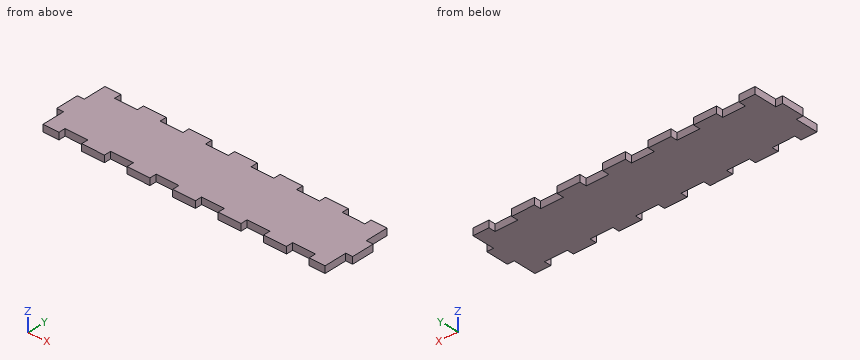
from build123d import *

# Parameters (mm, degrees)
F0_W     = 130
F0_H     = 30
F2_DEPTH = 3
F1_W     = 3
F1_H     = 10
F3_DEPTH = 25
F4_W     = 10
F4_H     = 3
F5_DEPTH = 25


with BuildPart() as f2:
    # F0 (on Top) → F2 (new body)
    with BuildSketch(Plane.XY):
        Rectangle(F0_W, F0_H)
    extrude(amount=F2_DEPTH)

    # F1 (on face) → F3 (cut)
    with BuildSketch(Plane.XY):
        with Locations((63.5, -10)):
            Rectangle(F1_W, F1_H)
        with Locations((63.5, 10)):
            Rectangle(F1_W, F1_H)
        with Locations((63.5, 30)):
            Rectangle(F1_W, F1_H)
        with Locations((63.5, 50)):
            Rectangle(F1_W, F1_H)
        with Locations((63.5, 70)):
            Rectangle(F1_W, F1_H)
        with Locations((63.5, 90)):
            Rectangle(F1_W, F1_H)
        with Locations((-63.5, -10)):
            Rectangle(F1_W, F1_H)
        with Locations((-63.5, 70)):
            Rectangle(F1_W, F1_H)
        with Locations((-63.5, 50)):
            Rectangle(F1_W, F1_H)
        with Locations((-63.5, 30)):
            Rectangle(F1_W, F1_H)
        with Locations((-63.5, 90)):
            Rectangle(F1_W, F1_H)
        with Locations((-63.5, 10)):
            Rectangle(F1_W, F1_H)
    extrude(amount=F3_DEPTH, mode=Mode.SUBTRACT)

    # F4 (on face) → F5 (cut)
    with BuildSketch(Plane.XY.offset(3)):
        with Locations((-50, -13.5)):
            Rectangle(F4_W, F4_H)
        with Locations((-30, -13.5)):
            Rectangle(F4_W, F4_H)
        with Locations((-10, -13.5)):
            Rectangle(F4_W, F4_H)
        with Locations((10, -13.5)):
            Rectangle(F4_W, F4_H)
        with Locations((30, -13.5)):
            Rectangle(F4_W, F4_H)
        with Locations((50, -13.5)):
            Rectangle(F4_W, F4_H)
        with Locations((30, 13.5)):
            Rectangle(F4_W, F4_H)
        with Locations((-50, 13.5)):
            Rectangle(F4_W, F4_H)
        with Locations((50, 13.5)):
            Rectangle(F4_W, F4_H)
        with Locations((-30, 13.5)):
            Rectangle(F4_W, F4_H)
        with Locations((70, 13.5)):
            Rectangle(F4_W, F4_H)
        with Locations((-10, 13.5)):
            Rectangle(F4_W, F4_H)
        with Locations((10, 13.5)):
            Rectangle(F4_W, F4_H)
    extrude(amount=-F5_DEPTH, mode=Mode.SUBTRACT)


solid = f2.part
Model file for the job. Use its own axes, mm. Coordinates: 2 decimals unless noted, no trailing zeros. Order: outer loops, then holes, each group sorted by start corner. A loop starts at its lowest first (then second) coordinate and runs counter-clockwise, first axis right, second up. Notation, with made-up numbers: M -29,43.25 L -11,43.25 A25 ccw -11,65.25 Z; hole C 72.5,27 d11. An arc over 180 degrees is marked long. Return JSON: item names as keys, results as strings.
1. Drill centre lines: probe 1 along X at (y, z) = (-11.75, 2.3); probe 2 along Y at (x, z) = (-52.5, 2.65). Where is each one in solid material? Low to high.
Ans:
{"probe 1": "-62 to 62", "probe 2": "-12 to 12"}
2. Saw through at A-A (x = -52). Give the cut face in (y, z), and give its area (3 significant figures).
Ans:
{"outline": "M -12,0 L 12,0 L 12,3 L -12,3 Z", "area": "72.0 mm^2"}
3. Flat gauge pins, fed straight in: pin 1 (1.5 mm diameter, centred on y = -14, z = 2, fed in from -X); pin 2 (0.9 mm diameter, centred on x = 31, z = 2, fed in from -Y); pin 3 (3 mm diameter, centred on x = -49.5, y = 4.5, fed in from -Z); pin 4 (1.5 mm diameter, centred on x = -49.5, z = 1.5, fed in from +Y). Where does each tip first touch, or does it go through?
Ans:
{"pin 1": "x = -62", "pin 2": "y = -12", "pin 3": "z = 0", "pin 4": "y = 12"}
4. Saw through at B-B (y = 8.5). Give the cut face in (x, z).
Ans:
{"outline": "M -62,0 L 62,0 L 62,3 L -62,3 Z"}
